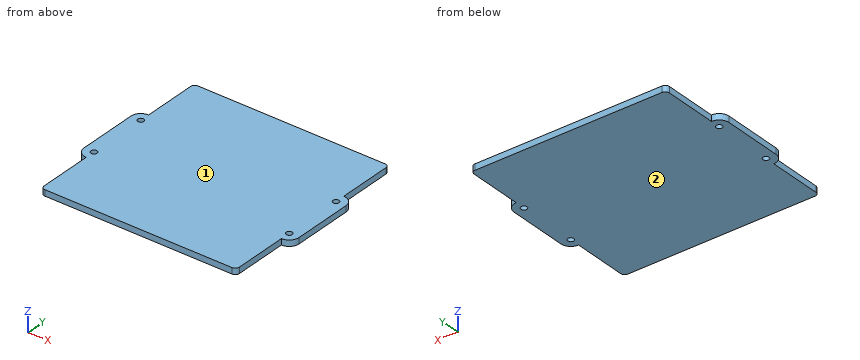
Autodesk Inventor part; units mm, degrees
ref_plane "YZ Plane" through (0, 0, 0) normal (1, 0, 0) x (0, 1, 0)
ref_plane "XZ Plane" through (0, 0, 0) normal (0, 1, 0) x (-1, 0, 0)
ref_plane "XY Plane" through (0, 0, 0) normal (0, 0, 1) x (1, 0, 0)
sketch "Sketch1" plane through (0, 0, 0) normal (0, 0, 1) x (1, 0, 0)
  line L0 (0, 0) -> (98, 0)
  line L1 (98, 0) -> (98, 98)
  line L2 (98, 98) -> (0, 98)
  line L3 (0, 98) -> (0, 0)
  line L4 (-5, 69) -> (103, 69)
  line L5 (103, 69) -> (103, 29)
  line L6 (103, 29) -> (-5, 29)
  line L7 (-5, 29) -> (-5, 69)
  dimension "d0" = 98
  dimension "d1" = 98
  dimension "d14" = 108
  dimension "d15" = 40
  dimension "d16" = 5
  dimension "d17" = 29
extrude "Extrusion1" add sketch "Sketch1" along normal blind 3
fillet "Fillet3" radius 2 4 edges at (0, 0, 1.5) (98, 0, 1.5) (0, 98, 1.5) (98, 98, 1.5)
fillet "Fillet9" radius 5 4 edges at (-5, 29, 1.5) (-5, 69, 1.5) (103, 29, 1.5) (103, 69, 1.5)
sketch "Sketch8" plane through (0, 0, 3) normal (0, 0, 1) x (1, 0, 0)
  arc A0 (0, 69) -> (-5, 64) centre (0, 64) ccw
  arc A1 (-5, 34) -> (0, 29) centre (0, 34) ccw
  arc A2 (98, 29) -> (103, 34) centre (98, 34) ccw
  arc A3 (103, 64) -> (98, 69) centre (98, 64) ccw
hole "Hole5" at (0, 34, 3) at (0, 64, 3) at (98, 34, 3) at (98, 64, 3) direction (0, 0, -1) diameter 3 end through all
properties part number "plastic_part_11"
Check sheet for the modelled part. Datum: model origin and axes. Units: mm. Face numbers are marked on the shaded views. Round coordinates to 2 decimals unless told otherwise and drop trailing zeros. Put each result on its own line as item: value.
(1) Mould release check, pull along Z, two halves, no side actions. Record for the marked faces 1 and 2: released by +Z, released by -Z, zero draft, split by the parting line, or undercut.
Values found:
face 1: released by +Z
face 2: released by -Z
(2) Material ranges on line 1 (X direction, y = 34, z = 1.5); line 2 (Y direction, x = 97.5, z = 0.55); line 3 (X direction, y = 19, z = 0.95), recorded low to high.
Values found:
line 1: x = -5 to -1.5, 1.5 to 96.5, 99.5 to 103
line 2: y = 0.68 to 32.59, 35.41 to 62.59, 65.41 to 97.32
line 3: x = 0 to 98
(3) Go/stop test with flat-tipped pins: pin 1 Ø0.9 at (y, z) = (77, 1) entering from +X; pin 2 Ø2.5 at (x, y) = (0, 34) entering from +Z; pin 3 Ø1.5 at (y, z) = (16.5, 1) entering from -X. Record where each tip stops, or that it passes through.
Values found:
pin 1: stops at x = 98
pin 2: passes through
pin 3: stops at x = 0
